Geometry check sheet. Reference: the model listing, model coordinates, mm. Face numbers are marked on the shaded views. A direction names the side the tool comes from. Coordinates: 2 decimals unless noted, no trailing zeros. Loops run counter-clockwise (first coordinate to the right, second up) from the corner with the lowest first, then second, coordinate; pieces in that order, holes last. Notation, with made-up numbers: (73, 66) - (132, 66) arc R5 cw to (132, 72) - close; hole circle Ø9 at (6, 85). An arc over 180 degrees is marked (long way). Write each question's results on one line, items separated by ' | '. Start each with the question number.
(1) Sectioned sample at C-C (z = -16). Enter the section's corners in (x, y).
(2) Mould release check, pull along X, two halves, no side actions. Record for the marked faces 3 and 4: pulls with the +X half, pulls with the -X half, needs draft (parallel to the pull), parting line crosses it, or undercut.
(3) Material ranges on probe 1 along Z at (x, y) = (23.85, 2.85); probe 2 along X at (y, z) = (2.75, -20.55); probe 3 along X at (y, z) = (2.5, -21.5), recorded low to high.
(4) Sectioned sample at D-D (x = 15). Enter the section's corners in (y, z).
(5) Go/stop test with a flat-tipped pin: pin 1 Ø4.5 at (x, z) = (23.85, -4.45) entering from -Y. Record where the tip stops, or that it passes through.
(6) Sectioned sample at B-B (y = 1.1). Enter the section's corners in (x, z).
(7) Access from +Z, -Z, +X, -X, +Y, -Y to the whole of each face (thin tool, end or side, straight path). Record for the marked faces 1 and 2.
(8) Sectioned sample at A-A (x = 6.15). State how many separate pieces and enclosed holes the cut face has, plus the area to 3 significant figures.
from build123d import *

# Parameters (mm, degrees)
SKETCH1_W           = 30
SKETCH1_H           = 25
SKETCH1_R           = 1.45
BOSS_EXTRUDE1_DEPTH = 3
SKETCH2_R           = 2.45
SKETCH2_R_2         = 1.45
BOSS_EXTRUDE2_DEPTH = 2
CUT_EXTRUDE1_DEPTH  = 2
FILLET1_R           = 1


with BuildPart() as part:
    # Sketch1 → Boss-Extrude1 (new body)
    with BuildSketch(Plane(origin=(0, 0, 0), x_dir=(1, 0, 0), z_dir=(0, 1, 0))):
        with Locations((15, 12.5)):
            Rectangle(SKETCH1_W, SKETCH1_H)
        with Locations(Location((6.15, 20.55, 0), (0, 0, 270))):
            Circle(SKETCH1_R, mode=Mode.SUBTRACT)
        with Locations(Location((23.85, 20.55, 0), (0, 0, 270))):
            Circle(SKETCH1_R, mode=Mode.SUBTRACT)
        with Locations(Location((6.15, 4.45, 0), (0, 0, 270))):
            Circle(SKETCH1_R, mode=Mode.SUBTRACT)
        with Locations(Location((23.85, 4.45, 0), (0, 0, 270))):
            Circle(SKETCH1_R, mode=Mode.SUBTRACT)
    extrude(amount=BOSS_EXTRUDE1_DEPTH)

    # Sketch2 → Boss-Extrude2 (add)
    # profile 1 of 4: a face of its own
    with BuildSketch(Plane(origin=(0, 3, 0), x_dir=(1, 0, 0), z_dir=(0, 1, 0))):
        with Locations(Location((6.15, 20.55, 0), (0, 0, 90))):
            Circle(SKETCH2_R)
        with Locations(Location((6.15, 20.55, 0), (0, 0, 270))):
            Circle(SKETCH2_R_2, mode=Mode.SUBTRACT)
    # profile 2 of 4: a face of its own
    with BuildSketch(Plane(origin=(0, 3, 0), x_dir=(1, 0, 0), z_dir=(0, 1, 0))):
        with Locations(Location((23.85, 20.55, 0), (0, 0, 90))):
            Circle(SKETCH2_R)
        with Locations(Location((23.85, 20.55, 0), (0, 0, 270))):
            Circle(SKETCH2_R_2, mode=Mode.SUBTRACT)
    # profile 3 of 4: a face of its own
    with BuildSketch(Plane(origin=(0, 3, 0), x_dir=(1, 0, 0), z_dir=(0, 1, 0))):
        with Locations(Location((6.15, 4.45, 0), (0, 0, 90))):
            Circle(SKETCH2_R)
        with Locations(Location((6.15, 4.45, 0), (0, 0, 270))):
            Circle(SKETCH2_R_2, mode=Mode.SUBTRACT)
    # profile 4 of 4: a face of its own
    with BuildSketch(Plane(origin=(0, 3, 0), x_dir=(1, 0, 0), z_dir=(0, 1, 0))):
        with Locations(Location((23.85, 4.45, 0), (0, 0, 90))):
            Circle(SKETCH2_R)
        with Locations(Location((23.85, 4.45, 0), (0, 0, 270))):
            Circle(SKETCH2_R_2, mode=Mode.SUBTRACT)
    extrude(amount=BOSS_EXTRUDE2_DEPTH)

    # Sketch3 → Cut-Extrude1 (cut)
    with BuildSketch(Plane.XZ):
        Polygon((7.679978213, -7.1), (9.209956427, -4.45), (7.679978213, -1.8), (4.620021787, -1.8), (3.090043573, -4.45), (4.620021787, -7.1), align=None)
        Polygon((25.379978213, -7.1), (26.909956427, -4.45), (25.379978213, -1.8), (22.320021787, -1.8), (20.790043573, -4.45), (22.320021787, -7.1), align=None)
        Polygon((25.379978213, -23.2), (26.909956427, -20.55), (25.379978213, -17.9), (22.320021787, -17.9), (20.790043573, -20.55), (22.320021787, -23.2), align=None)
        Polygon((7.679978213, -23.2), (9.209956427, -20.55), (7.679978213, -17.9), (4.620021787, -17.9), (3.090043573, -20.55), (4.620021787, -23.2), align=None)
    extrude(amount=-CUT_EXTRUDE1_DEPTH, mode=Mode.SUBTRACT)

    # Fillet1
    fillet1_edges = [part.edges().sort_by_distance(p)[0] for p in [
        (6.15, 3, -18.1),
        (23.85, 3, -18.1),
        (6.15, 3, -2),
        (23.85, 3, -2),
    ]]
    fillet(fillet1_edges, radius=FILLET1_R)


solid = part.part
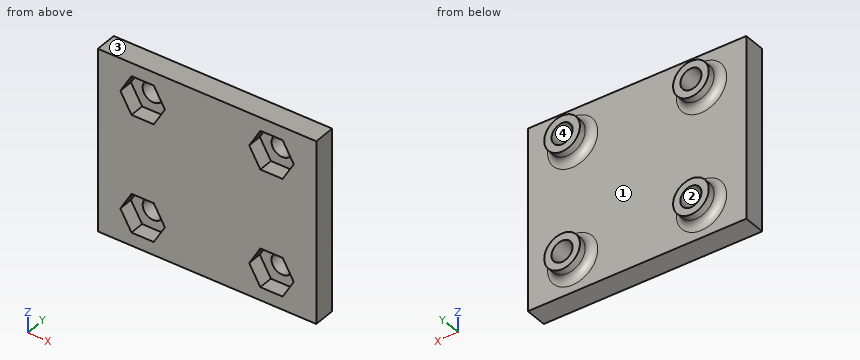
Outcome:
1) outline: (0, 0) - (30, 0) - (30, 3) - (0, 3) - close
2) face 3: needs draft | face 4: undercut
3) probe 1: z = -25 to -22, -19.1 to -5.9, -3 to 0 | probe 2: x = 0 to 4.7, 7.6 to 22.4, 25.3 to 30 | probe 3: x = 0 to 5.05, 7.25 to 22.75, 24.95 to 30
4) outline: (0, -25) - (3, -25) - (3, 0) - (0, 0) - close
5) pin 1: stops at y = 2
6) outline: (0, -25) - (30, -25) - (30, 0) - (0, 0) - close; hole (3.09, -20.55) - (4.62, -23.2) - (7.68, -23.2) - (9.21, -20.55) - (7.68, -17.9) - (4.62, -17.9) - close; hole (3.09, -4.45) - (4.62, -7.1) - (7.68, -7.1) - (9.21, -4.45) - (7.68, -1.8) - (4.62, -1.8) - close; hole (20.79, -20.55) - (22.32, -23.2) - (25.38, -23.2) - (26.91, -20.55) - (25.38, -17.9) - (22.32, -17.9) - close; hole (20.79, -4.45) - (22.32, -7.1) - (25.38, -7.1) - (26.91, -4.45) - (25.38, -1.8) - (22.32, -1.8) - close
7) face 1: +Y | face 2: +Y, -Y
8) separate pieces: 3 | enclosed holes: 0 | area: 56.9 mm2
